Design review of the part built by this model. Coordinates are the model's own, in mm. Face numbers are marked on the shaded views. A direction names the side the tool comes from. Round coordinates to 2 decimals unless told otherwise and drop trailing zeros. Write each loop counter-clockwise with the first axis right and the second up, starting at its lowest first coordinate (ties: lowest second). Pieces come first, ordered by that corner, then holes. Notation, with made-up numbers: M -31,44.25 L -12,44.25 A15 cw -12,73.25 Z; hole C -8.75,-31 d10. An arc over 180 degrees is marked long. Use CSV: the item, a comma, the result in double quotes.
from build123d import *

# Parameters (mm, degrees)
SKETCH7_R           = 1.65
SKETCH7_W           = 12
SKETCH7_H           = 12
BOSS_EXTRUDE2_DEPTH = 4
CUT_EXTRUDE6_DEPTH  = 3
FILLET3_R           = 3
SKETCH10_W          = 12
SKETCH10_H          = 12
CUT_EXTRUDE7_DEPTH  = 2


with BuildPart() as part:
    # Sketch7 → Boss-Extrude2 (new body)
    # profile 1 of 3: a face of its own
    with BuildSketch(Plane.XY):
        Polygon((-6, -10), (-6, -6), (-6, -2), (-16, -2), (-16, -10), align=None)
        with Locations((-11, -6)):
            Circle(SKETCH7_R, mode=Mode.SUBTRACT)
    # profile 2 of 3: a face of its own
    with BuildSketch(Plane.XY):
        Rectangle(SKETCH7_W, SKETCH7_H)
    # profile 3 of 3: a face of its own
    with BuildSketch(Plane.XY):
        Polygon((6, 6), (6, 2), (16, 2), (16, 10), (6, 10), align=None)
        with Locations((11, 6)):
            Circle(SKETCH7_R, mode=Mode.SUBTRACT)
    extrude(amount=BOSS_EXTRUDE2_DEPTH)

    # Sketch9 → Cut-Extrude6 (cut)
    with BuildSketch(Plane.XY.offset(4)):
        Polygon((-11, -2.824573519), (-13.75, -4.41228676), (-13.75, -7.58771324), (-11, -9.175426481), (-8.25, -7.58771324), (-8.25, -4.41228676), align=None)
        Polygon((11, 2.824573519), (13.75, 4.41228676), (13.75, 7.58771324), (11, 9.175426481), (8.25, 7.58771324), (8.25, 4.41228676), align=None)
    extrude(amount=-CUT_EXTRUDE6_DEPTH, mode=Mode.SUBTRACT)

    # Fillet3
    fillet3_edges = [part.edges().sort_by_distance(p)[0] for p in [
        (-16, -2, 2),
        (-6, 6, 2),
        (6, 10, 2),
        (16, 10, 2),
        (16, 2, 2),
        (6, -6, 2),
        (-6, -10, 2),
        (-16, -10, 2),
    ]]
    fillet(fillet3_edges, radius=FILLET3_R)

    # Sketch10 → Cut-Extrude7 (cut)
    with BuildSketch(Plane(origin=(0, 0, 0), x_dir=(-1, 0, 0), z_dir=(0, 0, -1))):
        Rectangle(SKETCH10_W, SKETCH10_H)
    extrude(amount=-CUT_EXTRUDE7_DEPTH, mode=Mode.SUBTRACT)


solid = part.part
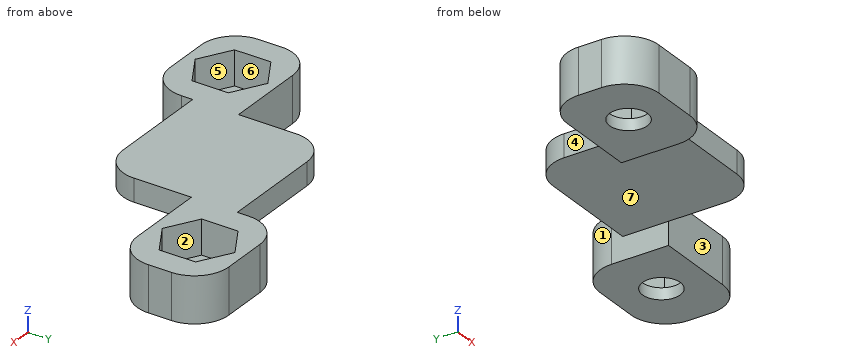
1) Machinability: for the marked faces 1, 2 and 3, which of the approach directions +Z, -Z, +X, -X, +Y, -Y give a long, thin tool a straight path to every point of the face, cutting with its end or side? Answer none if there is none.
Answers:
face 1,"+Z, -Z, -X, +Y"
face 2,"+Z"
face 3,"+Z, -Z, +X, -Y"
2) Add section C-C on y = -3.75. Write out the cut boundary in (x, z).
Answers:
outline,"M -15.73,0 L -6,0 L -6,2 L 5.9,2 L 5.9,4 L -9.4,4 L -9.4,1 L -12.6,1 L -12.6,4 L -15.73,4 Z"
3) For pin 1 Ø5.5 at (x, y) = (-11, -6) entering from -Z; pin 2 Ø1.5 at (y, z) = (2.5, 2) entering from -X; pin 3 Ø0.6 at (x, z) = (1, 2.5) entering from +Y; pin 4 Ø2 at (x, z) = (-2.5, 2.5) entering from -Y, all flat-tipped, find the tip position at first contact; note any pin that passes through.
Answers:
pin 1,"z = 0"
pin 2,"x = -6"
pin 3,"y = 6"
pin 4,"y = -6"
4) Wall thickness on line 1 along Y through (x, z) = (11, 0.4); line 2 along Y through (x, z) = (-11, 0.3); line 3 along X through (y, z) = (6, 0.7): over which ranges is each line inside the solid? List them lowest first. Write a range as [from, to].
Answers:
line 1,"[2, 4.35], [7.65, 10]"
line 2,"[-10, -7.65], [-4.35, -2]"
line 3,"[6, 9.35], [12.65, 16]"
5) Add section D-D on x = -2. Write out the cut boundary in (y, z), then the cut area to 3 significant figures.
Answers:
outline,"M -6,2 L 6,2 L 6,4 L -6,4 Z"
area,"24.0 mm²"
6) Add section A-A on z = 2.45. Give the number of separate pieces and of enclosed holes in the cut face, then the cut area to 3 significant figures.
Answers:
separate pieces,"1"
enclosed holes,"2"
area,"236 mm²"
7) The part is to be moulded in two halves that separate along X. For the marked faces 4, 5, 6 and 7, say which applies: released by +X, released by -X, zero draft, split by the parting line, or undercut.
Answers:
face 4,"released by -X"
face 5,"undercut"
face 6,"undercut"
face 7,"zero draft"
8) Add section B-B on y = -6.5. Write out the cut boundary in (x, z), then the cut area to 3 significant figures.
Answers:
outline,"M -16,0 L -12.57,0 L -12.57,1 L -13.75,1 L -13.75,4 L -16,4 Z; M -9.43,0 L -6,0 L -6,4 L -8.25,4 L -8.25,1 L -9.43,1 Z"
area,"20.4 mm²"
